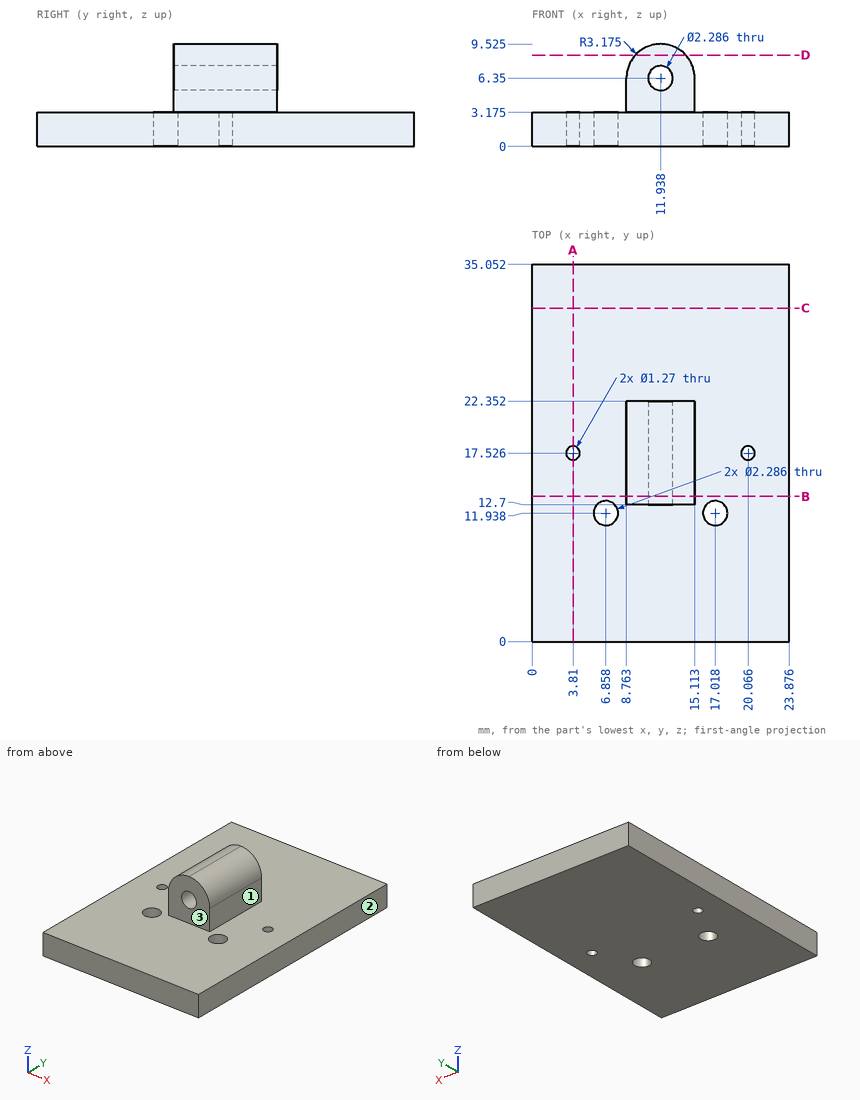
Geometry: see drawing. Coordinates: mm, zero at the bounding-box minimum. A direction names the side the tool comes from. Coordinates: 2 decimals unless noted, no trailing zeros. Loops run counter-clockwise (first coordinate to the right, second up) from the corner with the lowest first, then second, coordinate; pieces in that order, holes last.
Q1. Set-up query: the marked faces 1, 2 and 3. Return all of +Z, -Z, +X, -X, +Y, -Y with unobstructed straight access to the full face (end or side cutting, diameter ignored); none if empty.
Q2. Cut plane A-A (x = 3.81). Output: boundary loops of the cut face in (y, z) (3 decimals), then the cut area to 3 significant figures.
Q3. Material intervals for line 1 (X direction, y = 17, z = 1); line 2 (Y direction, x = 3.81, z = 0.9); line 3 (Z direction, x = 22.75, y = 16) (3 decimals), sorted ascending.
Q4. Cut plane C-C (y = 31). Output: boundary loops of the cut face in (x, z) (3 decimals), then the cut area to 3 significant figures.
Q5. Cut plane B-B (y = 13.5). Output: boundary loops of the cut face in (x, z) (3 decimals), then the cut area to 3 significant figures.
Q6. Contact query for flat-ended pins moving along their axis: pin 1 (2.5 mm diameter, centred on y = 16.5, z = 4.5, fed in from +X); pin 2 (2.5 mm diameter, centred on y = 19, z = 4.5, fed in from -X); pin 3 (3 mm diameter, centred on x = 13, z = 7, fed in from -Y). Output: stop coordinate, or through.
Q7. Cut plane D-D (z = 8.5). Output: boundary loops of the cut face in (x, y).
Working result:
1. face 1: +Z, +X, +Y, -Y
1. face 2: +Z, -Z, +X, +Y, -Y
1. face 3: +Z, +X, -X, -Y
2. outline: (0, 0) - (16.891, 0) - (16.891, 3.175) - (0, 3.175) - close; (18.161, 0) - (35.052, 0) - (35.052, 3.175) - (18.161, 3.175) - close
2. area: 107 mm2
3. line 1: x = 0 to 3.45, 4.17 to 19.71, 20.42 to 23.88
3. line 2: y = 0 to 16.89, 18.16 to 35.05
3. line 3: z = 0 to 3.175
4. outline: (0, 0) - (23.876, 0) - (23.876, 3.175) - (0, 3.175) - close
4. area: 75.8 mm2
5. outline: (0, 0) - (23.876, 0) - (23.876, 3.175) - (15.113, 3.175) - (15.113, 6.35) arc R3.175 ccw to (8.763, 6.35) - (8.763, 3.175) - (0, 3.175) - close; hole circle Ø2.286 at (11.938, 6.35)
5. area: 108 mm2
6. pin 1: stops at x = 15.11
6. pin 2: stops at x = 8.76
6. pin 3: stops at y = 12.7
7. outline: (9.6, 12.7) - (14.27, 12.7) - (14.27, 22.35) - (9.6, 22.35) - close
